Autodesk Inventor part; units mm, degrees
ref_plane "Work Plane2" through (25.4, 0, 0) normal (1, 0, 0) x (0, 1, 0)
ref_plane "XZ Plane" through (0, 0, 0) normal (0, 1, 0) x (-1, 0, 0)
ref_plane "XY Plane" through (0, 0, 0) normal (0, 0, 1) x (1, 0, 0)
sketch "Sketch1" plane through (0, 0, 0) normal (0, 1, 0) x (-1, 0, 0)
  line L0 (-78, -86) -> (78, -86)
  line L1 (78, -86) -> (78, 86)
  line L2 (78, 86) -> (-78, 86)
  line L3 (-78, 86) -> (-78, -86)
  line L4 (-78, -86) -> (78, 86) construction
  line L5 (78, -86) -> (-78, 86) construction
  point P0 (0, 0)
  dimension "d0" = 156
  dimension "d1" = 172
extrude "Extrusion1" add sketch "Sketch1" along normal blind 3.175
sketch "Sketch2" plane through (0, 3.175, 0) normal (0, 1, 0) x (1, 0, 0)
  line L0 (65.3, 73.3) -> (14.5, 73.3)
  line L1 (14.5, 73.3) -> (14.5, -73.3)
  line L2 (14.5, -73.3) -> (65.3, -73.3)
  line L3 (65.3, -73.3) -> (65.3, 73.3)
  line L4 (78, 86) -> (-78, 86)
  line L5 (78, -86) -> (78, 86)
  point P0 (0, 0)
  point P1 (65.3, 0)
  point P2 (39.9, 73.3)
  point P3 (39.9, -73.3)
  dimension "d4" = 50.8
  dimension "d5" = 12.7
  dimension "d45" = 38.1
hole "Hole1" at (39.9, 3.175, -73.3) at (39.9, 3.175, 73.3) at (65.3, 3.175, -73.3) at (14.5, 3.175, -73.3) at (14.5, 3.175, 73.3) at (65.3, 3.175, 73.3) direction (0, -1, 0) diameter 4.5 end through all
mirror "Mirror1" about plane through (0, 0, 0) normal (1, 0, 0) of "Hole1"
sketch "Sketch3" plane through (-78, 0, -86) normal (-1, 0, 0) x (0, 0, 1)
  line L0 (0, 0) -> (172, 0)
  line L1 (172, 0) -> (172, 3.175)
  line L2 (0, 3.175) -> (172, 3.175)
  line L3 (0, 0) -> (0, 3.175)
  point P0 (86, 0)
extrude "Extrusion2" add sketch "Sketch3" along normal blind 25.4
sketch "Sketch6" plane through (78, 0, 86) normal (1, 0, 0) x (0, 0, -1)
  line L0 (0, 0) -> (172, 0)
  line L1 (172, 0) -> (172, 3.175)
  line L2 (0, 3.175) -> (172, 3.175)
  line L3 (0, 0) -> (0, 3.175)
  point P0 (86, 0)
extrude "Extrusion3" add sketch "Sketch6" along normal blind 63.5
sketch "Sketch4" plane through (0, 3.175, 0) normal (0, 1, 0) x (1, 0, 0)
  line L0 (-81.9624, 82.0312) -> (-81.9624, 64.5687)
  circle A0 centre (-65.3, 73.3) radius 2.25
  line L1 (-103.4, -86) -> (-103.4, 86)
  point P0 (0, 0)
  point P1 (-81.9624, 73.3)
  dimension "d16" = 17.4625
  dimension "d17" = 21.4376
hole "Hole2" at (-81.9624, 3.175, -64.5687) at (-81.9624, 3.175, -82.0312) direction (0, -1, 0) diameter 5.3 end through all
ref_plane "Work Plane2" through (25.4, 0, 0) normal (1, 0, 0) x (0, 1, 0)
mirror "Mirror3" about plane through (0, 0, 0) normal (0, 0, 1) of "Hole2"
mirror "Mirror4" about plane through (25.4, 0, 0) normal (1, 0, 0) of "Hole2", "Mirror3"
sketch "Sketch5" plane through (0, 3.175, 0) normal (0, 1, 0) x (1, 0, 0)
  line L0 (-76.4, 33) -> (76.4, 33)
  line L1 (76.4, 33) -> (76.4, -33)
  line L2 (76.4, -33) -> (-76.4, -33)
  line L3 (-76.4, -33) -> (-76.4, 33)
  line L4 (-76.4, 33) -> (76.4, -33) construction
  line L5 (76.4, 33) -> (-76.4, -33) construction
  line L6 (-103.4, -86) -> (-103.4, 86)
  line L7 (76.4, 11) -> (-76.4, 11)
  line L8 (-76.4, 11) -> (-76.4, -11)
  line L9 (-76.4, -11) -> (76.4, -11)
  line L10 (76.4, -11) -> (76.4, 11)
  line L11 (76.4, 11) -> (-76.4, -11) construction
  line L12 (-76.4, 11) -> (76.4, -11) construction
  point P0 (0, 0)
  point P1 (-103.4, -84)
  point P2 (-103.4, 84)
  dimension "d26" = 66
  dimension "d35" = 27
  dimension "d36" = 22
hole "Hole3" at (76.4, 3.175, -33) at (76.4, 3.175, 33) at (-76.4, 3.175, -33) at (-76.4, 3.175, 33) at (-76.4, 3.175, 11) at (-76.4, 3.175, -11) at (76.4, 3.175, 11) at (76.4, 3.175, -11) direction (0, -1, 0) diameter 4.5 end through all
sketch "Sketch7" plane through (0, 3.175, 0) normal (0, 1, 0) x (1, 0, 0)
  line L0 (141.5, 86) -> (141.5, -86)
  line L1 (103.4, 60.6) -> (141.5, 60.6)
  line L2 (141.5, 60.6) -> (141.5, -60.6)
  line L3 (141.5, -60.6) -> (103.4, -60.6)
  line L4 (103.4, -60.6) -> (103.4, 60.6)
  line L5 (103.4, 60.6) -> (141.5, -60.6) construction
  line L6 (141.5, 60.6) -> (103.4, -60.6) construction
  point P0 (0, 0)
  point P1 (141.5, 84)
  point P2 (141.5, -84)
  point P3 (122.45, 0)
  point P4 (122.45, 0)
  dimension "d40" = 121.2
  dimension "d41" = 38.1
extrude "Extrusion4" cut sketch "Sketch7" against normal through all
fillet "Fillet2" radius 2 8 edges at (141.5, 1.5875, 60.6) (141.5, 1.5875, -60.6) (141.5, 1.5875, -86) (103.4, 1.5875, -60.6) (103.4, 1.5875, 60.6) (141.5, 1.5875, 86) (-103.4, 1.5875, 86) (-103.4, 1.5875, -86)
sketch "Sketch8" plane through (0, 3.175, 0) normal (0, 1, 0) x (1, 0, 0)
  line L0 (28.25, -22.75) -> (-28.25, -22.75)
  line L1 (-28.25, -22.75) -> (-28.25, 22.75)
  line L2 (-28.25, 22.75) -> (28.25, 22.75)
  line L3 (28.25, 22.75) -> (28.25, -22.75)
  line L4 (28.25, -22.75) -> (-28.25, 22.75) construction
  line L5 (-28.25, -22.75) -> (28.25, 22.75) construction
  point P0 (0, 0)
  dimension "d46" = 56.5
  dimension "d47" = 45.5
extrude "Extrusion5" cut sketch "Sketch8" against normal blind 1.6
ref_plane "Work Plane1" through (0, 0, 0) normal (1, 0, 0) x (0, 1, 0)
properties part number "Battery_Base"
Build history of the part. All positions in model axes, mm. A direction names the side the tool comes from. Coordinates: 2 decimals unless noted, no trailing zeros. Order: outer loops, then holes, each group sorted by start corner. A loop starts at its lowest first (then second) coordinate and runs counter-clockwise, first axis right, second up. Notation, with made-up numbers: (-20, 75) - (-2, 75) arc R31 ccw to (-2, 108) - close; hole circle Ø6 at (75, 64.25). An arc over 180 degrees is marked (long way). Put each result on its own line as item: value.
1. Saw through at B-B (z = 19). Write the cut outline in (x, y) (3 decimals).
Answer sheet:
outline: (-103.4, 0) - (103.4, 0) - (103.4, 3.175) - (28.25, 3.175) - (28.25, 1.575) - (-28.25, 1.575) - (-28.25, 3.175) - (-103.4, 3.175) - close
2. Saw through at C-C (x = -3). Write the cut outline in (y, z) (3 decimals).
Answer sheet:
outline: (0, -86) - (3.175, -86) - (3.175, -22.75) - (1.575, -22.75) - (1.575, 22.75) - (3.175, 22.75) - (3.175, 86) - (0, 86) - close
3. Drop flat-ended pins along their axis: P1, Ø3.5, axis at x = -14.5, z = 73.3, coming from the -Y side; P2, Ø0.5, axis at y = 2, z = 1.5, coming from the +X side. Give the stop position or say it passes through.
Answer sheet:
P1: passes through
P2: stops at x = 103.4
4. Saw through at D-D (y = 1). Give the number of separate pieces and of enclosed holes in the cut face, and give its area (3 significant figures).
Answer sheet:
separate pieces: 1
enclosed holes: 28
area: 37,000 mm^2
5. Probe line 1 along X through (y, z) = (1.9, -11); line 2 along Z through (x, y) = (17.5, 2.5); line 3 along X through (y, z) = (0.7, 33). List the from-to ranges inside material, lowest first. Write a range as [from, to].
Answer sheet:
line 1: x = [-103.4, -78.65], [-74.15, -28.25], [28.25, 74.15], [78.65, 103.4]
line 2: z = [-86, -22.75], [22.75, 86]
line 3: x = [-103.4, -78.65], [-74.15, 74.15], [78.65, 103.4]
6. Tool access for faces 3 (the face through (0, 1.575, 0)), 4 (the face through (15.36, 1.57, 75.38)): list every direction of +Z, -Z, +X, -X, +Y, -Y with a clear straight run to the whole face (end or side of a thin tool).
Answer sheet:
face 3: +Y
face 4: +Y, -Y
7. Pull direction X, two halves, no side cores. Call faces 1 (the face through (-75.54, 1.57, -30.92)), 2 (the face through (45, 3.175, 1)): pulls with the +X half, pulls with the -X half, needs draft (parallel to the pull), parting line crosses it, or undercut.
Answer sheet:
face 1: undercut
face 2: needs draft
8. Saw through at A-A (x = 124). Write the cut outline in (y, z) (3 decimals).
Answer sheet:
outline: (0, -86) - (3.175, -86) - (3.175, -60.6) - (0, -60.6) - close; (0, 60.6) - (3.175, 60.6) - (3.175, 86) - (0, 86) - close
